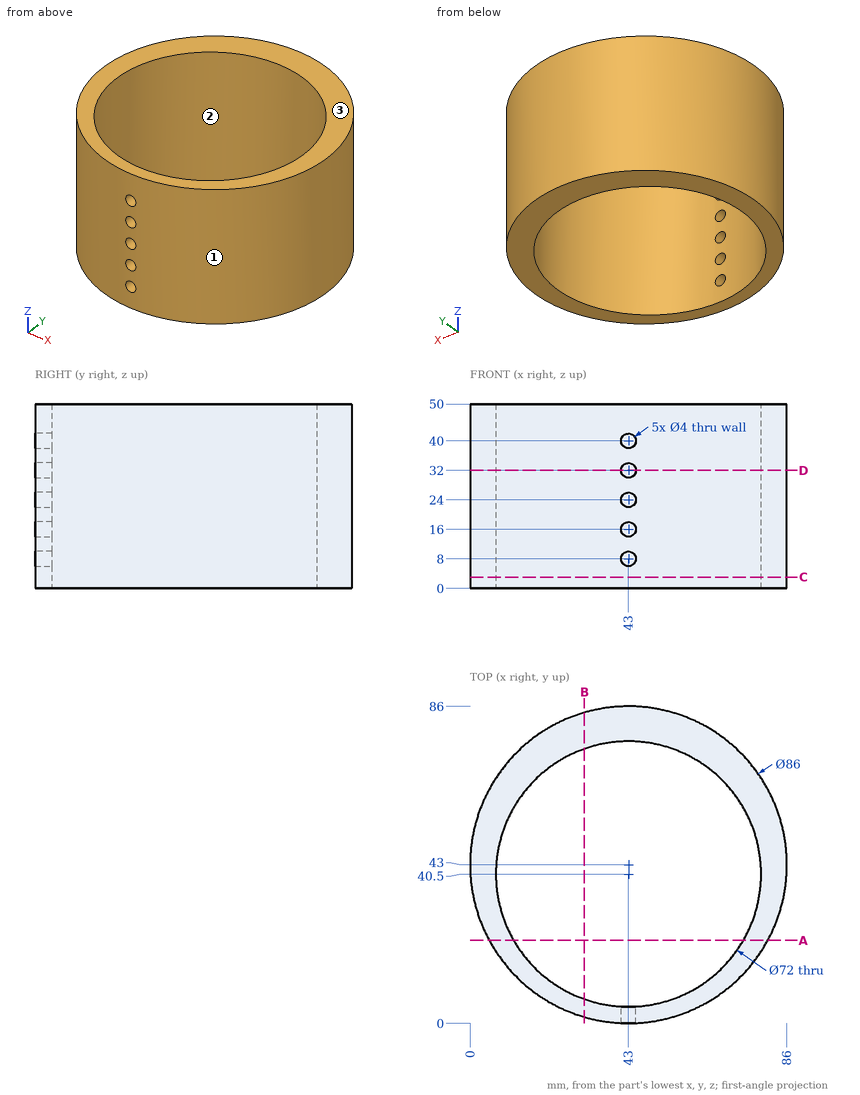
Design review of the part shown in the three views and the two pictorial views. Dimensions are in mm from the part's minimum x, y and z. Round coordinates to 2 decimals unless told otherwise and drop trailing zeros. Order: outer loops, then holes, each group sorted by start corner. A loop starts at its lowest first (then second) coordinate and runs counter-clockwise, first axis right, second up. Notation, with made-up numbers: (-39, 78) -> (-33, 78) arc R23 ccw to (-33, 99) -> close; hole circle Ø10 at (45.5, 43.25). An arc over 180 degrees is marked (long way). Write item = value, one per line. Start each with the question number.
1) The part is to be moulded in two halves that separate along X. For the marked faces 1, 2 and 3, say which applies: +X half, -X half, draft (parallel to the pull), parting line (faces both ways), or undercut.
2) Take a section at B-B on x = 31. State the section outline as (y, z) points, plus the area to 3 significant figures.
3) Insertion check: pin 1 (5 mm diameter, centred on x = 21, y = 64, fed in from -Z); pin 2 (1 mm diameter, centred on y = 59.5, z = 25, fed in from -X); pin 3 (6.5 mm diameter, centred on x = 43, z = 16, fed in from +Y); pin 4 (6 mm diameter, centred on x = 68.5, z = 39.5, fed in from -Y). Each pin has a flat end and moves straight along its axis. Give the tip position at first contact, or say it passes through.
4) To check wall thickness, follow line 1 (Y direction, x = 47.5, z = 15); line 2 (X direction, y = 12.5, z = 16); line 3 (X direction, y = 3, z = 40). State the ranges of each line that lie inside material, in increasing order. Write a range as from..to.
5) Take a section at A-A on y = 22.5. State the section outline as (x, z) points, plus the area to 3 significant figures.
6) Take a section at C-C on z = 3. State the section outline as (x, y) points, plus the area to 3 significant figures.
7) Take a section at D-D on z = 32. State the section outline as (x, y) points, plus the area to 3 significant figures.
Verdict:
q1.face_1 = parting line
q1.face_2 = undercut
q1.face_3 = draft
q2.outline = (1.71, 0) -> (6.56, 0) -> (6.56, 50) -> (1.71, 50) -> close; (74.44, 0) -> (84.29, 0) -> (84.29, 50) -> (74.44, 50) -> close
q2.area = 735 mm2
q3.pin_1 = through
q3.pin_2 = 3.09
q3.pin_3 = 86
q3.pin_4 = 6.36
q4.line_1 = 0.24..4.78, 76.22..85.76
q4.line_2 = 12.69..20.37, 65.63..73.31
q4.line_3 = 27.22..41, 45..58.78
q5.outline = (5.2, 0) -> (11.82, 0) -> (11.82, 50) -> (5.2, 50) -> close; (74.18, 0) -> (80.8, 0) -> (80.8, 50) -> (74.18, 50) -> close
q5.area = 662 mm2
q6.outline = circle Ø86 at (43, 43); hole circle Ø72 at (43, 40.5)
q6.area = 1,740 mm2
q7.outline = (41, 0.05) -> (41, 4.56) arc R36 cw (long way) to (45, 4.56) -> (45, 0.05) arc R43 ccw (long way) to start
q7.area = 1,720 mm2
